```python
from build123d import *

# Parameters (mm, degrees)
SKETCH1_R           = 6.1
BOSS_EXTRUDE1_DEPTH = 3
SKETCH2_R           = 1.6
CUT_EXTRUDE1_DEPTH  = 4
BOSS_EXTRUDE2_DEPTH = 1.5
BOSS_EXTRUDE3_DEPTH = 3


with BuildPart() as part:
    # Sketch1 → Boss-Extrude1 (new body)
    with BuildSketch(Plane(origin=(0, 0, 0), x_dir=(1, 0, 0), z_dir=(0, 1, 0))):
        with BuildLine():
            Line((-10, -10), (10, -10))
            Line((10, -10), (10, 10))
            ThreePointArc((10, 10), (0, 20), (-10, 10))
            Line((-10, 10), (-10, -10))
        make_face()
        with Locations((0, 10)):
            Circle(SKETCH1_R, mode=Mode.SUBTRACT)
    extrude(amount=BOSS_EXTRUDE1_DEPTH)

    # Sketch2 → Cut-Extrude1 (cut, through all)
    with BuildSketch(Plane(origin=(0, 3, 0), x_dir=(1, 0, 0), z_dir=(0, 1, 0))):
        with Locations((-5, -6)):
            Circle(SKETCH2_R)
        with Locations((5, -6)):
            Circle(SKETCH2_R)
    extrude(amount=-CUT_EXTRUDE1_DEPTH, mode=Mode.SUBTRACT)

    # Sketch4 → Boss-Extrude2 (add, symmetric)
    with BuildSketch(Plane(origin=(0, 0, 0), x_dir=(0, 0, -1), z_dir=(1, 0, 0))):
        Polygon((-10, 3), (-10, 9), (2, 3), align=None)
    extrude(amount=BOSS_EXTRUDE2_DEPTH, both=True)

    # Sketch5 → Boss-Extrude3 (add)
    with BuildSketch(Plane(origin=(0, 0, 0), x_dir=(1, 0, 0), z_dir=(0, 1, 0))):
        Polygon((-10, -10), (-12, -10), (-10, -6.535898385), align=None)
        Polygon((10, -10), (12, -10), (10, -6.535898385), align=None)
    extrude(amount=BOSS_EXTRUDE3_DEPTH)


solid = part.part
```
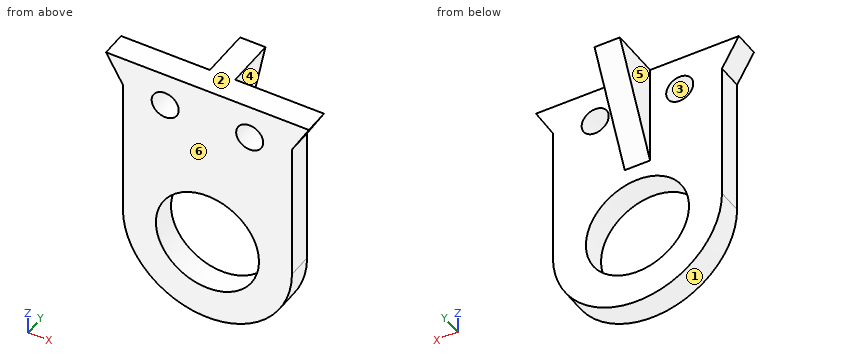
For this review, take the finished solid that the model builds, in its own axes (mm). Face numbers are marked on the shaded views. A direction names the side the tool comes from. Round coordinates to 2 decimals unless told otherwise and drop trailing zeros. Write each loop counter-clockwise with the first axis right and the second up, starting at its lowest first coordinate (ties: lowest second). Pieces come first, ordered by that corner, then holes. Notation, with made-up numbers: (10.5, 70) -> (44.5, 70) arc R24 ccw to (44.5, 99) -> close; hole circle Ø4 at (33.25, 72.5). An arc over 180 degrees is marked (long way). Use one line per item in the form item = value.
1) Mouldability with a two-part tool opening along X and no side actions: class the marked faces 1, 2 and 3 as +X half, -X half, draft (parallel to the pull), parting line (faces both ways), or undercut.
Found:
face_1 = parting line
face_2 = draft
face_3 = undercut
2) Take a section at C-C, the plane y = 1. Write out the cut boundary in (x, z).
Found:
outline = (-12, 10) -> (-10, 6.54) -> (-10, -10) arc R10 ccw to (10, -10) -> (10, 6.54) -> (12, 10) -> close; hole circle Ø3.2 at (-5, 6); hole circle Ø12.2 at (0, -10); hole circle Ø3.2 at (5, 6)
3) To check wall thickness, follow L1, parallel to X at y = 1.65, z = 6; L2, parallel to Z at x = -5, y = 2.35; L3, parallel to Z at x = 0, y = 2.1. State the ranges of each line that lie inside material, in increasing order. Write a range as from..to.
Found:
L1 = -10..-6.6, -3.4..3.4, 6.6..10
L2 = -18.66..-13.49, -6.51..4.4, 7.6..10
L3 = -20..-16.1, -3.9..10
4) Clearance check with flat-ended pins moving along their axes: pin 1 (4 mm diameter, centred on x = -4, z = 0, fed in from +Y); pin 2 (2.5 mm diameter, centred on y = 1.5, z = -1, fed in from -X); pin 3 (0.9 mm diameter, centred on y = 1, z = 2, fed in from +X). State where each tip first meets the part, or that it passes through.
Found:
pin_1 = 3
pin_2 = -10
pin_3 = 10
5) Tool access review of the marked faces 4, 5 and 6: name each direction out of +Z, -Z, +X, -X, +Y, -Y from which nothing blocks a thin tool from reaching the whole face with its end or side.
Found:
face_4 = +Z, -Z, +X, +Y
face_5 = +Z, -Z, -X, +Y
face_6 = +Z, -Z, +X, -X, -Y
6) Take a section at A-A, the plane z = 6. Write out the cut boundary in (x, y).
Found:
outline = (-10, 0) -> (-6.6, 0) -> (-6.6, 3) -> (-10, 3) -> close; (-3.4, 0) -> (3.4, 0) -> (3.4, 3) -> (1.5, 3) -> (1.5, 7) -> (-1.5, 7) -> (-1.5, 3) -> (-3.4, 3) -> close; (6.6, 0) -> (10, 0) -> (10, 3) -> (6.6, 3) -> close
7) Take a section at D-D, the plane z = -8. Write out the cut boundary in (x, y), and give its area (3 significant figures).
Found:
outline = (-10, 0) -> (-5.76, 0) -> (-5.76, 3) -> (-10, 3) -> close; (5.76, 0) -> (10, 0) -> (10, 3) -> (5.76, 3) -> close
area = 25.4 mm2
8) Take a section at B-B, the plane x = 0. Write out the cut boundary in (y, z).
Found:
outline = (0, -20) -> (3, -20) -> (3, -16.1) -> (0, -16.1) -> close; (0, -3.9) -> (3, -3.9) -> (3, -2) -> (9, 10) -> (0, 10) -> close
